Autodesk Inventor part; units mm, degrees
ref_plane "YZ Plane" through (0, 0, 0) normal (1, 0, 0) x (0, 1, 0)
ref_plane "XZ Plane" through (0, 0, 0) normal (0, 1, 0) x (-1, 0, 0)
ref_plane "XY Plane" through (0, 0, 0) normal (0, 0, 1) x (1, 0, 0)
sketch "スケッチ1" plane through (0, 0, 0) normal (0, 0, 1) x (1, 0, 0)
  line L0 (0, 0) -> (27.1, 0) construction
  line L1 (0, -4) -> (27.1, -4)
  line L2 (27.1, 4) -> (0, 4)
  arc A0 (0, 4) -> (0, -4) centre (0, 0) ccw
  arc A1 (27.1, -4) -> (27.1, 4) centre (27.1, 0) ccw
  circle A2 centre (0, 0) radius 1.6
  circle A3 centre (27.1, 0) radius 2.6
  circle A4 centre (27.1, 0) radius 5
  point P0 (13.55, 0)
  dimension "d0" = 27.1
  dimension "d1" = 4
  dimension "d2" = 3.2
  dimension "d3" = 5.2
  dimension "d6" = 10
extrude "押し出し1" add sketch "スケッチ1" along normal blind 3
sketch "スケッチ3" plane through (0, 0, 0) normal (0, 0, 1) x (1, 0, 0)
  circle A0 centre (0, 0) radius 4
  circle A1 centre (0, 0) radius 1.6
  dimension "d7" = 8
  dimension "d10" = 3.2
extrude "押し出し2" add sketch "スケッチ3" against normal blind 0.5
sketch "スケッチ4" plane through (0, 0, 0) normal (0, 0, 1) x (1, 0, 0)
  circle A0 centre (0, 0) radius 1.6
  circle A1 centre (0, 0) radius 2.5
  dimension "d11" = 5
  dimension "d12" = 3.2
extrude "押し出し3" add sketch "スケッチ4" against normal blind 3.7
sketch "スケッチ5" plane through (0, 0, 3) normal (0, 0, 1) x (1, 0, 0)
  circle A0 centre (0, 0) radius 1.6
  arc A1 (0, 4) -> (0, -4) centre (0, 0) ccw
  line L0 (0, 3.2332) -> (2.8, 1.6166)
  line L1 (2.8, 1.6166) -> (2.8, -1.6166)
  line L2 (2.8, -1.6166) -> (0, -3.2332)
  line L3 (0, -3.2332) -> (-2.8, -1.6166)
  line L4 (-2.8, -1.6166) -> (-2.8, 1.6166)
  line L5 (-2.8, 1.6166) -> (0, 3.2332)
  dimension "d15" = 5.6
extrude "押し出し4" cut sketch "スケッチ5" against normal blind 1.5
fillet "フィレット1" radius 2 2 edges at (24.1, 4, 1.5) (24.1, -4, 1.5)
properties part number "link_long"
Design review of the part built by this model. Coordinates are the model's own, in mm. A direction names the side the tool comes from. Round coordinates to 2 decimals unless told otherwise and drop trailing zeros. Order: outer loops, then holes, each group sorted by start corner. A loop starts at its lowest first (then second) coordinate and runs counter-clockwise, first axis right, second up. Notation, with made-up numbers: (25, -11.75) - (63, -11.75) arc R9 cw to (63, -3.75) - close; hole circle Ø9 at (48.5, 20). An arc over 180 degrees is marked (long way). Return JSON: item names as keys, results as strings.
Q1. Machinability: for faces 1 (the flat face through (12, -4, 1)), 2 (the flat face through (12, 4, 1)), 3 (the flat face through (-1.38, -2.436, 2.26)), which of the approach directions +Z, -Z, +X, -X, +Y, -Y give a long, thin tool a straight path to every point of the face, cutting with its end or side? Answer none if there is none.
Computed values:
{"face 1": "+Z, -Z, -X, -Y", "face 2": "+Z, -Z, -X, +Y", "face 3": "+Z"}
Q2. Consider section C-C on z = -1.25. Write out the cut boundary in (x, y).
Computed values:
{"outline": "circle Ø5 at (0, 0); hole circle Ø3.2 at (0, 0)"}
Q3. Consider section B-B on y = 0. Write out the cut boundary in (x, z), plus the area to 3 significant figures.
Computed values:
{"outline": "(-4, -0.5) - (-2.5, -0.5) - (-2.5, -3.7) - (-1.6, -3.7) - (-1.6, 1.5) - (-2.8, 1.5) - (-2.8, 3) - (-4, 3) - close; (1.6, -3.7) - (2.5, -3.7) - (2.5, -0.5) - (4, -0.5) - (4, 0) - (24.5, 0) - (24.5, 3) - (2.8, 3) - (2.8, 1.5) - (1.6, 1.5) - close; (29.7, 0) - (32.1, 0) - (32.1, 3) - (29.7, 3) - close", "area": "87.7 mm2"}
Q4. The part is to be moulded in two halves that separate along X. For faces 4 (the flat face through (2.8, 0, 2)), 5 (the flat face through (1.42, -2.414, 2.26)), 6 (the flat face through (2, 2, -0.5)), 7 (the cylindrical face through (24.02, 4.07, 1.52)), say which applies: pulls with the +X half, pulls with the -X half, needs draft (parallel to the pull), parting line crosses it, or undercut.
Computed values:
{"face 4": "undercut", "face 5": "undercut", "face 6": "needs draft", "face 7": "pulls with the -X half"}
Q5. For pin 1 Ø3.5 at (x, z) = (16, 1) entering from +Y; pin 2 Ø2.5 at (x, y) = (0, 0) entering from -Z; pin 3 Ø1.5 at (x, z) = (13, 2) entering from -Y; pin 4 Ø5 at (x, y) = (22, -1) entering from -Z, all flat-tipped, find the tip position at first contact; note any pin that passes through.
Computed values:
{"pin 1": "stops at y = 4", "pin 2": "passes through", "pin 3": "stops at y = -4", "pin 4": "stops at z = 0"}
Q6. Consider section D-D on x = 6.5. Write out the cut boundary in (y, z).
Computed values:
{"outline": "(-4, 0) - (4, 0) - (4, 3) - (-4, 3) - close"}
Q7. Wall thickness on L1, parallel to Y at x = 27.1, z = 2.1; L2, parallel to X at y = 2, z = 2.5; L3, parallel to X at y = -1.5, z = 2: over which ranges is each line inside the solid? List them lowest first. Write a range as [from, to].
Computed values:
{"L1": "y = [-5, -2.6], [2.6, 5]", "L2": "x = [-3.46, -2.14], [2.14, 25.44], [28.76, 31.68]", "L3": "x = [-3.71, -2.8], [2.8, 24.98], [29.22, 31.87]"}
Q8. Consider section A-A on x = 27.1. Write out the cut boundary in (y, z).
Computed values:
{"outline": "(-5, 0) - (-2.6, 0) - (-2.6, 3) - (-5, 3) - close; (2.6, 0) - (5, 0) - (5, 3) - (2.6, 3) - close"}
